Job drawing, mm, ordinate dimensions from the low corner. One solid piece. Round coordinates to 2 decimals unless told otherwise and drop trailing zeros. Write each loop counter-clockwise with the first axis right and the second up, starting at its lowest first coordinate (ties: lowest second). Pieces come first, ordered by that corner, then holes. Notation, with made-up numbers: (68, -0.75) - (81, -0.75) arc R33 cw to (81, 33.25) - close; hole circle Ø10 at (-21.5, -24.5). An arc over 180 degrees is marked (long way). Write each question's results on one line, items separated by ' | '.
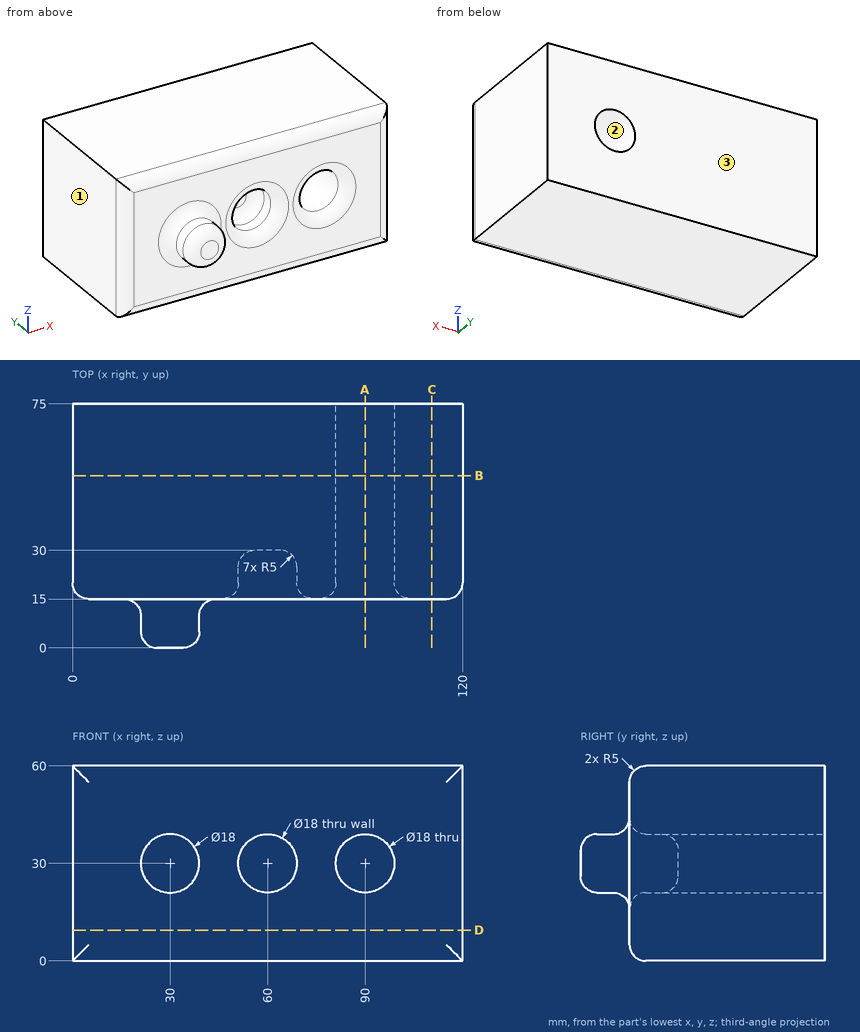
(1) Slice it at A-A, the plane x = 90. Write the cut outline in (y, z), and give its area (3 significant figures).
Worked answers:
outline: (15, 5) arc R5 ccw to (20, 0) - (75, 0) - (75, 21) - (20, 21) arc R5 ccw to (15, 16) - close; (15, 44) arc R5 ccw to (20, 39) - (75, 39) - (75, 60) - (20, 60) arc R5 ccw to (15, 55) - close | area: 2,500 mm2
(2) Slice it at D-D, the plane z = 9.5. Write the cut outline in (x, y).
Worked answers:
outline: (0, 20) arc R5 ccw to (5, 15) - (115, 15) arc R5 ccw to (120, 20) - (120, 75) - (0, 75) - close
(3) Slice it at C-C, the plane x = 110.5. Write the cut outline in (y, z), and give its area (3 significant figures).
Worked answers:
outline: (15, 5) arc R5 ccw to (20, 0) - (75, 0) - (75, 60) - (20, 60) arc R5 ccw to (15, 55) - close | area: 3,590 mm2
(4) Drill centre lines: probe 1 along X at (y, z) = (23.5, 30); probe 2 along Z at (x, y) = (90, 52.5); probe 3 along X at (y, z) = (31, 30). Where is each one in solid material? Low to high. Write a range as [from, to].
Worked answers:
probe 1: x = [0, 51], [69, 81], [99, 120] | probe 2: z = [0, 21], [39, 60] | probe 3: x = [0, 81], [99, 120]
(5) Flat gauge pins, fed straight in: pin 1 Ø1.5 at (x, z) = (86.5, 45.5) entering from -Y; pin 2 Ø2.5 at (x, z) = (59.5, 32) entering from -Y. Where does each tip first touch, or does it go through?
Worked answers:
pin 1: stops at y = 15 | pin 2: stops at y = 30
(6) Slice it at B-B, the plane y = 53. Write the cut outline in (x, z), and give its area (3 significant figures).
Worked answers:
outline: (0, 0) - (120, 0) - (120, 60) - (0, 60) - close; hole circle Ø18 at (90, 30) | area: 6,950 mm2
(7) Two-plate mould, pull along X, no slides. Class the marked faces 1, 2 and 3: released by +X, released by -X, zero draft, split by the parting line, or undercut.
Worked answers:
face 1: released by -X | face 2: undercut | face 3: zero draft
